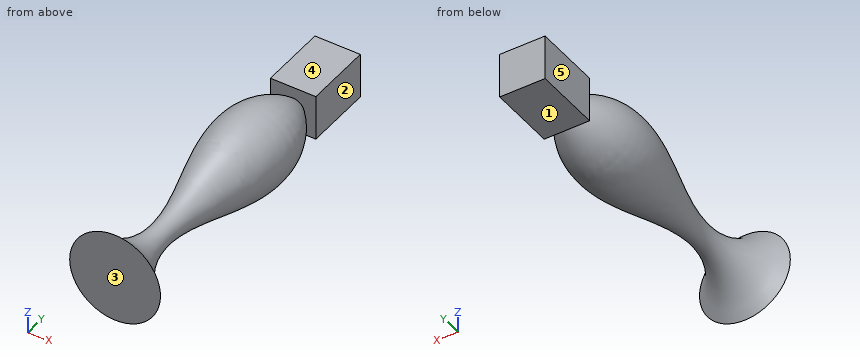
from build123d import *

# Parameters (mm, degrees)
SKETCH10_W          = 101.6
SKETCH10_H          = 101.6
BOSS_EXTRUDE5_DEPTH = 152.4


with BuildPart() as part:
    # Sketch1 → Revolve3 (revolve)
    with BuildSketch(Plane.XY):
        with BuildLine():
            Line((0, 0), (0, -152.4))
            Line((0, -152.4), (-101.6, -152.4))
            add(Edge.make_bspline(
                [(-101.6, -152.4), (112.233734467, 26.074070803), (-211.807575975, 256.743639399), (-25.4, 457.2)],
                knots=[0, 0, 0, 0, 1, 1, 1, 1], degree=3))
            Line((-25.4, 457.2), (0, 457.2))
            Line((0, 457.2), (0, 0))
        make_face()
    revolve(axis=Axis((0, 0, 0), (0, 1, 0)))

    # Sketch10 → Boss-Extrude5 (add)
    with BuildSketch(Plane(origin=(0, 457.2, 0), x_dir=(1, 0, 0), z_dir=(0, 1, 0))):
        Rectangle(SKETCH10_W, SKETCH10_H)
    extrude(amount=BOSS_EXTRUDE5_DEPTH)


solid = part.part
Geometry check sheet. Reference: the model listing, model coordinates, mm. Face numbers are marked on the shaded views. A direction names the side the tool comes from. Give positions to 0.01 mm unless a question says otherwise; leave off trailing zeros. Write each loop counter-clockwise with the first axis right and the second up, starting at its lowest first coordinate (ties: lowest second). Pieces come first, ordered by that corner, then holes.
1) Cross-section at A-A (y = 475). Record the boundary of the cut face in (x, z).
Values follow:
outline: (-50.8, -50.8) - (50.8, -50.8) - (50.8, 50.8) - (-50.8, 50.8) - close
2) Thickness scan on line 1 (X direction, y = 545, z = -32); line 2 (Y direction, x = -71, z = 53). Record the ranges inside material, lowest first.
Values follow:
line 1: x = -50.8 to 50.8
line 2: y = -152.4 to -140.87
3) Cross-section at B-B (z = -42). Count the separate pieces of the cut face and the enclosed holes in it, plus the area to 3 significant figures.
Values follow:
separate pieces: 3
enclosed holes: 0
area: 59,100 mm2
4) Go/stop test with flat-tipped pins: pin 1 Ø12 at (y, z) = (273, 46) entering from +X; pin 2 Ø1 at (y, z) = (-73, 2.5) entering from -X; pin 3 Ø10 at (y, z) = (478, -15.5) entering from +X. Record where each tip stops, or that it passes through.
Values follow:
pin 1: stops at x = 73.84
pin 2: stops at x = -39.99
pin 3: stops at x = 50.8
5) Set-up check for the marked faces 1, 2, 3, 4 and 5: record each of +Z, -Z, +X, -X, +Y, -Y from which the full face is reachable in a straight line by a thin tool's end or side.
Values follow:
face 1: -Z, +X, -X, +Y
face 2: +Z, -Z, +X, +Y
face 3: +Z, -Z, +X, -X, -Y
face 4: +Z, +X, -X, +Y
face 5: +Z, -Z, -X, +Y
